Geometry check sheet. Reference: the model listing, model coordinates, mm. Coordinates: 2 decimals unless noted, no trailing zeros. Write each loop counter-clockwise with the first axis right and the second up, starting at its lowest first coordinate (ties: lowest second). Pieces come first, ordered by that corner, then holes. Notation, with made-up numbers: (-22.5, 89.5) -> (18.5, 89.5) arc R20 ccw to (18.5, 119.5) -> close; hole circle Ø9 at (27.25, -4). An arc over 180 degrees is marked (long way). Answer in a Markdown table with one row per item. Add a question column.
Q1. Thickness scan on line 1 (X direction, y = 25, z = 11); line 2 (Y direction, x = -1, z = 0); line 3 (Y direction, x = -6.5, z = 0). Record the ranges inside material, lowest first.
Q2. Release check for a two-part mould opening along Z. For faces 1 (the face through (-15.5, -19.4, 19.4)), 2 (the face through (-12.176, 32.825, 17.073)), 3 (the face through (-0.188, -7.509, 23.846)) record: pulls with the +Z half, pulls with the -Z half, needs draft (parallel to the pull), parting line crosses it, or undercut.
Q3. Section check C-C, the plane x = 11.5. Record the boundary of the cut face in (y, z).
Q4. Section check B-B, the plane z = 0. Record the boundary of the cut face in (x, y), and give its area (3 significant figures).
Q5. Gauge pin test, flat ends, axial feed: P1, Ø1.5, axis at x = -9, z = 19, coming from the -Y side; P2, Ø3, axis at x = 6, z = -24.5, coming from the -Y side; P3, Ø3, axis at x = 6, z = -9, coming from the +Y side (3 decimals). Record the tip position at first contact, or that the pin passes through.
Q6. Section check D-D, the plane x = -6. Record the boundary of the cut face in (y, z), and give its area (3 significant figures).
Q7. Section check A-A, the plane y = 0. Record the boundary of the cut face in (x, z), and give its area (3 significant figures).
```python
from build123d import *

# Parameters (mm, degrees)
SKETCH2_W           = 4.289378808
SKETCH2_H           = 4.50384775
BOSS_EXTRUDE1_DEPTH = 1


with BuildPart() as part:
    # Sketch1 → Revolve2 (revolve)
    with BuildSketch(Plane.XY, mode=Mode.PRIVATE) as revolve2_sk:
        with BuildLine():
            Line((-15.5, 37), (-8.94427191, 37))
            ThreePointArc((-8.94427191, 37), (0, 33), (8.94427191, 37))
            Line((8.94427191, 37), (15.5, 37))
            Line((15.5, 37), (15.5, 27.1))
            ThreePointArc((15.5, 27.1), (14.88492424, 25.61507576), (13.4, 25))
            Line((13.4, 25), (-13.4, 25))
            ThreePointArc((-13.4, 25), (-14.88492424, 25.61507576), (-15.5, 27.1))
            Line((-15.5, 27.1), (-15.5, 37))
        make_face()
    revolve(revolve2_sk.sketch.rotate(Axis((-15.146387833, 0, 0), (1, 0, 0)), 90), axis=Axis((-15.146387833, 0, 0), (1, 0, 0)))

    # Sketch2 → Boss-Extrude1 (add)
    with BuildSketch(Plane(origin=(15.5, 0, 0), x_dir=(0, 0, -1), z_dir=(1, 0, 0))):
        with Locations((0, 31.871583754)):
            Rectangle(SKETCH2_W, SKETCH2_H)
    extrude(amount=BOSS_EXTRUDE1_DEPTH)


solid = part.part
```
Calculated:
| question | item | result |
|---|---|---|
| 1 | line 1 | x = -15.5 to 15.5 |
| 1 | line 2 | y = -33.04 to -25, 25 to 33.04 |
| 1 | line 3 | y = -34.91 to -25, 25 to 34.91 |
| 2 | face 1 | needs draft |
| 2 | face 2 | parting line crosses it |
| 2 | face 3 | undercut |
| 3 | outline | circle Ø74 at (0, 0); hole circle Ø50 at (0, 0) |
| 4 | outline | (-15.5, -37) -> (-8.94, -37) arc R12 cw to (8.94, -37) -> (15.5, -37) -> (15.5, -27.1) arc R2.1 ccw to (13.4, -25) -> (-13.4, -25) arc R2.1 ccw to (-15.5, -27.1) -> close; (-15.5, 27.1) arc R2.1 ccw to (-13.4, 25) -> (13.4, 25) arc R2.1 ccw to (15.5, 27.1) -> (15.5, 29.62) -> (16.5, 29.62) -> (16.5, 34.12) -> (15.5, 34.12) -> (15.5, 37) -> (8.94, 37) arc R12 cw to (-8.94, 37) -> (-15.5, 37) -> close |
| 4 | area | 646 mm² |
| 5 | P1 | stops at y = -32.19 |
| 5 | P2 | stops at y = -26.39 |
| 5 | P3 | stops at y = 34.535 |
| 6 | outline | circle Ø69.22 at (0, 0); hole circle Ø50 at (0, 0) |
| 6 | area | 1,800 mm² |
| 7 | outline | (-15.5, -37) -> (-8.94, -37) arc R12 cw to (8.94, -37) -> (15.5, -37) -> (15.5, -27.1) arc R2.1 ccw to (13.4, -25) -> (-13.4, -25) arc R2.1 ccw to (-15.5, -27.1) -> close; (-15.5, 27.1) arc R2.1 ccw to (-13.4, 25) -> (13.4, 25) arc R2.1 ccw to (15.5, 27.1) -> (15.5, 37) -> (8.94, 37) arc R12 cw to (-8.94, 37) -> (-15.5, 37) -> close |
| 7 | area | 641 mm² |
